Geometry check sheet. Reference: the model listing, model coordinates, mm. A direction names the side the tool comes from. Give positions to 0.01 mm unless a question says otherwise; leave off trailing zeros. Order: outer loops, then holes, each group sorted by start corner. A loop starts at its lowest first (then second) coordinate and runs counter-clockwise, first axis right, second up.
from build123d import *

# Parameters (mm, degrees)
PAD_DEPTH       = 50
SKETCH001_R     = 1.7
POCKET_DEPTH    = 10.001
SKETCH003_R     = 1.55
POCKET001_DEPTH = 8.001


with BuildPart() as part:
    # Sketch → Pad (new body)
    with BuildSketch(Plane.XZ):
        with BuildLine():
            Line((0, 0), (0, 8))
            Line((0, 8), (10, 8))
            Line((10, 8), (10, 6))
            Line((10, 6), (7, 6))
            ThreePointArc((7, 6), (3.464466, 4.535534), (2, 1))
            Line((2, 1), (2, 0))
            Line((2, 0), (0, 0))
        make_face()
    extrude(amount=PAD_DEPTH)

    # Sketch001 (on Face1 of Pad) → Pocket (cut, through all)
    with BuildSketch(Plane(origin=(0, 0, 0), x_dir=(0, 0, -1), z_dir=(-1, 0, 0))):
        with Locations((-4, 5)):
            Circle(SKETCH001_R)
        with Locations((-4, 45)):
            Circle(SKETCH001_R)
    extrude(amount=-POCKET_DEPTH, mode=Mode.SUBTRACT)

    # Sketch003 (on Face5 of Pocket) → Pocket001 (cut, through all)
    with BuildSketch(Plane(origin=(0, 0, 8), x_dir=(-1, 0, 0), z_dir=(0, 0, 1))):
        with Locations((-5, 38)):
            Circle(SKETCH003_R)
        with Locations((-5, 12)):
            Circle(SKETCH003_R)
    extrude(amount=-POCKET001_DEPTH, mode=Mode.SUBTRACT)


solid = part.part
Item 1: Sectioned sample at B-B (y = -12). Enter the section's corners in (x, z).
Reported:
outline: (0, 0) - (2, 0) - (2, 1) arc R5 cw to (3.45, 4.52) - (3.45, 8) - (0, 8) - close; (6.55, 5.98) arc R5 cw to (7, 6) - (10, 6) - (10, 8) - (6.55, 8) - close
Item 2: Sectioned sample at A-A (z = 4). Enter the section's corners in (x, y).
Reported:
outline: (0, -50) - (3, -50) - (3, -46.7) - (0, -46.7) - close; (0, -43.3) - (3, -43.3) - (3, -6.7) - (0, -6.7) - close; (0, -3.3) - (3, -3.3) - (3, 0) - (0, 0) - close
Item 3: Sectioned sample at C-C (x = 1.5). Enter the section's corners in (y, z).
Reported:
outline: (-50, 0) - (0, 0) - (0, 8) - (-50, 8) - close; hole circle Ø3.4 at (-45, 4); hole circle Ø3.4 at (-5, 4)
Item 4: Scan lines: L1, parallel to Y at x = 5, z = 7; L2, parallel to Z at x = 1.7, y = -5; L3, parallel to Y at x = 4.25, z = 5.5. Record each from-to range of solid material in increasing order.
Reported:
L1: y = -50 to -39.55, -36.45 to -13.55, -10.45 to 0
L2: z = 0 to 2.3, 5.7 to 8
L3: y = -50 to -45.8, -44.2 to -39.36, -36.64 to -13.36, -10.64 to -5.8, -4.2 to 0
Item 5: Gauge pin test, flat ends, axial feed: pin 1 (4 mm diameter, centred on x = 4.5, y = -34.5, fed in from -Z); pin 2 (3.5 mm diameter, centred on x = 8, y = -20, fed in from -Z); pin 3 (4 mm diameter, centred on y = -37.5, z = 3.5, fed in from +X). Record the tip position at first contact, or that the pin passes through.
Reported:
pin 1: stops at z = 3.18
pin 2: stops at z = 5.94
pin 3: stops at x = 4.4
Item 6: Sectioned sample at D-D (z = 6.5). Enter the section's corners in (x, y).
Reported:
outline: (0, -50) - (10, -50) - (10, 0) - (0, 0) - close; hole circle Ø3.1 at (5, -38); hole circle Ø3.1 at (5, -12)
Item 7: Draft check along X on faces 3 (the flat face through (2, -24.6, 0.5)), 4 (the cylindrical face through (3.522, -38.466, 6.671)), 5 (the flat face through (1, -25, 0)), 6 (the flat face through (0, -25, 4)). Enter one of: released by +X, released by -X, zero draft, split by the parting line, or undercut.
Reported:
face 3: released by +X
face 4: undercut
face 5: zero draft
face 6: released by -X
Item 8: Set-up check for faces 1 (the flat face through (9, -25, 6)), 2 (the cylindrical face through (3.522, -12.466, 6.671)): record each of +Z, -Z, +X, -X, +Y, -Y from which the full face is reachable in a straight line by a thin tool's end or side.
Reported:
face 1: -Z, +X, +Y, -Y
face 2: +Z, -Z
